Design review of the part shown in the three views and the two pictorial views. Dimensions are in mm from the part's minimum x, y and z. Give positions to 0.01 mm unless a question says otherwise; leave off trailing zeros. Loops run counter-clockwise (first coordinate to the right, second up) from the corner with the lowest first, then second, coordinate; pieces in that order, holes last. Notation, with made-up numbers: (-19.75, 79) - (5.25, 79) arc R22 ccw to (5.25, 102) - close; hole circle Ø2 at (86, 18). An arc over 180 degrees is marked (long way). Answer as a JSON object with one key per item and string values.
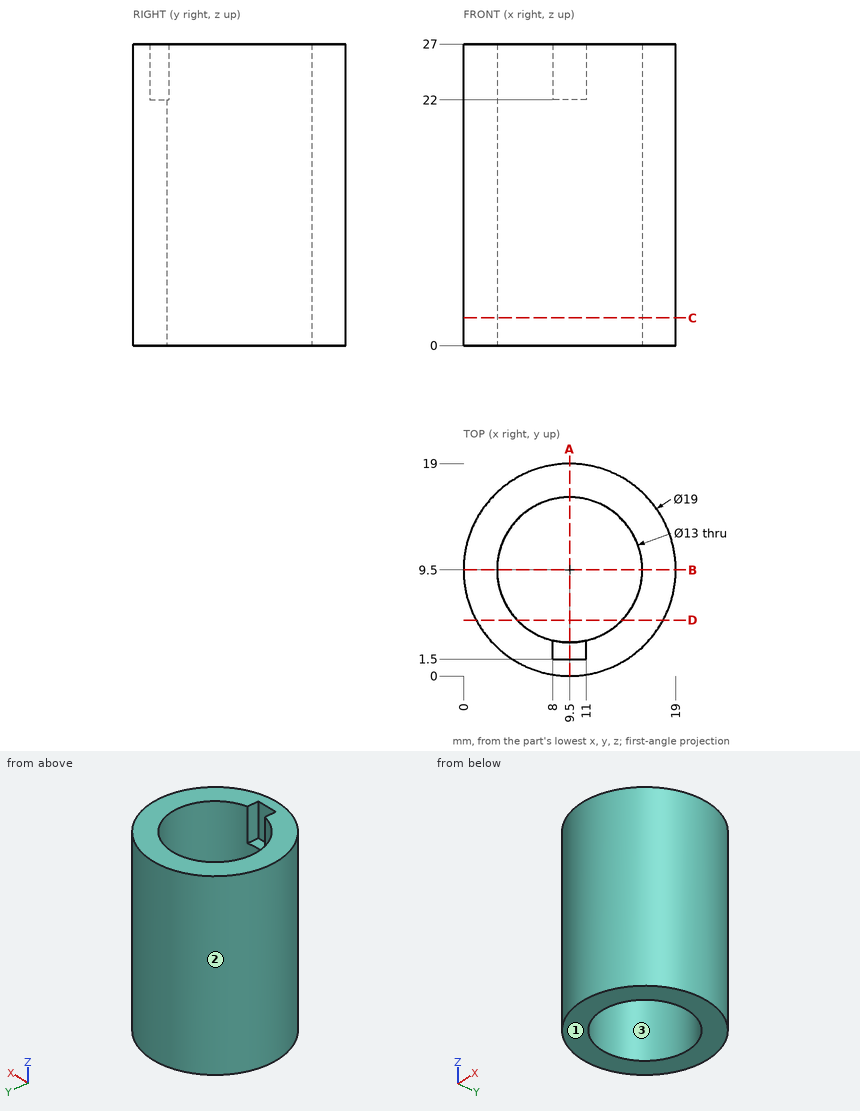
Q1. To check wall thickness, follow probe 1 along Y at (x, z) = (9.5, 20.5); probe 2 along X at (y, z) = (11, 5.75); probe 3 along Y at (x, z) = (3.5, 7.5). State the ranges of each line that lie inside material, in increasing order. Write a range as [from, to].
Results:
{"probe 1": "y = [0, 3], [16, 19]", "probe 2": "x = [0.12, 3.18], [15.82, 18.88]", "probe 3": "y = [2.13, 7], [12, 16.87]"}
Q2. Consider section A-A, the plane x = 9.5. State the section outline as (y, z) points, plus the area to 4 significant figures.
Results:
{"outline": "(0, 0) - (3, 0) - (3, 22) - (1.5, 22) - (1.5, 27) - (0, 27) - close; (16, 0) - (19, 0) - (19, 27) - (16, 27) - close", "area": "154.5 mm^2"}
Q3. The part is to be moulded in two halves that separate along X. For the marked faces 1, 2 and 3, say which applies: +X half, -X half, draft (parallel to the pull), parting line (faces both ways), or undercut.
Results:
{"face 1": "draft", "face 2": "parting line", "face 3": "undercut"}
Q4. Consider section C-C, the plane z = 2.5. State the section outline as (x, y) points.
Results:
{"outline": "circle Ø19 at (9.5, 9.5); hole circle Ø13 at (9.5, 9.5)"}
Q5. Consider section B-B, the plane y = 9.5. State the section outline as (x, z) points.
Results:
{"outline": "(0, 0) - (3, 0) - (3, 27) - (0, 27) - close; (16, 0) - (19, 0) - (19, 27) - (16, 27) - close"}
Q6. Clearance check with flat-ended pins moving along their axes: pin 1 Ø1 at (x, z) = (15, 23) entering from -Y; pin 2 Ø5 at (y, z) = (15, 9) entering from -X; pin 3 Ø5 at (x, z) = (15.5, 9.5) entering from +Y. State where each tip first meets the part, or that it passes through.
Results:
{"pin 1": "stops at y = 1.42", "pin 2": "stops at x = 0.49", "pin 3": "stops at y = 18.33"}
Q7. Consider section D-D, the plane y = 5. State the section outline as (x, z) points, plus the area to 3 significant figures.
Results:
{"outline": "(1.13, 0) - (4.81, 0) - (4.81, 27) - (1.13, 27) - close; (14.19, 0) - (17.87, 0) - (17.87, 27) - (14.19, 27) - close", "area": "199 mm^2"}
